```python
from build123d import *


with BuildPart() as part:
    # Sketch1 → Revolve-Thin1 (revolve)
    with BuildSketch(Plane(origin=(0, 0, 0), x_dir=(0, 0, -1), z_dir=(1, 0, 0))):
        with BuildLine():
            Line((0, 30), (0, 26))
            Line((0, 26), (12, 8.862223919))
            ThreePointArc((12, 8.862223919), (10.506209129, 4.542549196), (10, 0))
            Line((10, 0), (9.5, 0))
            ThreePointArc((9.5, 0), (9.986787691, 4.509912766), (11.42472682, 8.812075766))
            Line((11.42472682, 8.812075766), (-0.5, 25.842350606))
            Line((-0.5, 25.842350606), (-0.5, 30))
            Line((-0.5, 30), (0, 30))
        make_face()
    revolve(axis=Axis((0, 0, -12), (0, 0, 1)))


solid = part.part
```
Work out the finished part from the listing and answer in its coordinate system (mm). Round coordinates to 2 decimals unless told otherwise and drop trailing zeros. Order: outer loops, then holes, each group sorted by start corner. A loop starts at its lowest first (then second) coordinate and runs counter-clockwise, first axis right, second up.
Q1. A cutting plane is placed at A-A, the plane x = 0. Determine the outline of the cut face in (y, z), then the cut area to 3 significant figures.
Solution:
outline: (-30, 0) - (-26, 0) - (-8.86, -12) arc R20.63 cw to (8.86, -12) - (26, 0) - (30, 0) - (30, 0.5) - (25.84, 0.5) - (8.81, -11.42) arc R21.13 ccw to (-8.81, -11.42) - (-25.84, 0.5) - (-30, 0.5) - close
area: 34.1 mm2
Q2. Find the intervals of material crossed by line 1 along Z through (x, y) = (27, -9.5); line 2 along X through (y, z) = (-4.5, -6); line 3 along X through (y, z) = (-4, -0.5), in increasing order.
Solution:
line 1: z = 0 to 0.5
line 2: x = -16.84 to -15.94, 15.94 to 16.84
line 3: x = -24.97 to -24.08, 24.08 to 24.97
Q3. A cutting plane is placed at C-C, the plane z = -7. Determine the outline of the cut face in (x, y).
Solution:
outline: circle Ø32.01 at (0, 0); hole circle Ø30.26 at (0, 0)
Q4. The mould has two halves that part along Y. Classify faces 1 (the cylindrical face through (-1.32, -29.97, 0.25)), 2 (the flat face through (-25, -9, 0.5)), 3 (the conical face through (9.64, -2.14, -10.68)): pulls with the +Y half, pulls with the -Y half, needs draft (parallel to the pull), parting line crosses it, or undercut.
Solution:
face 1: parting line crosses it
face 2: needs draft
face 3: undercut
Q5. Given pin 1 Ø6 at (x, z) = (-0.5, -6.5) entering from +Y; pin 2 Ø6 at (x, z) = (1.5, -10) entering from -Y; pin 3 Ø12 at (x, y) = (11.5, -15) entering from +Z, each flat-ended and moving along its own axis, determine where each tip first touches the part or whether it passes through.
Solution:
pin 1: stops at y = 21
pin 2: stops at y = -15.94
pin 3: stops at z = -0.16
